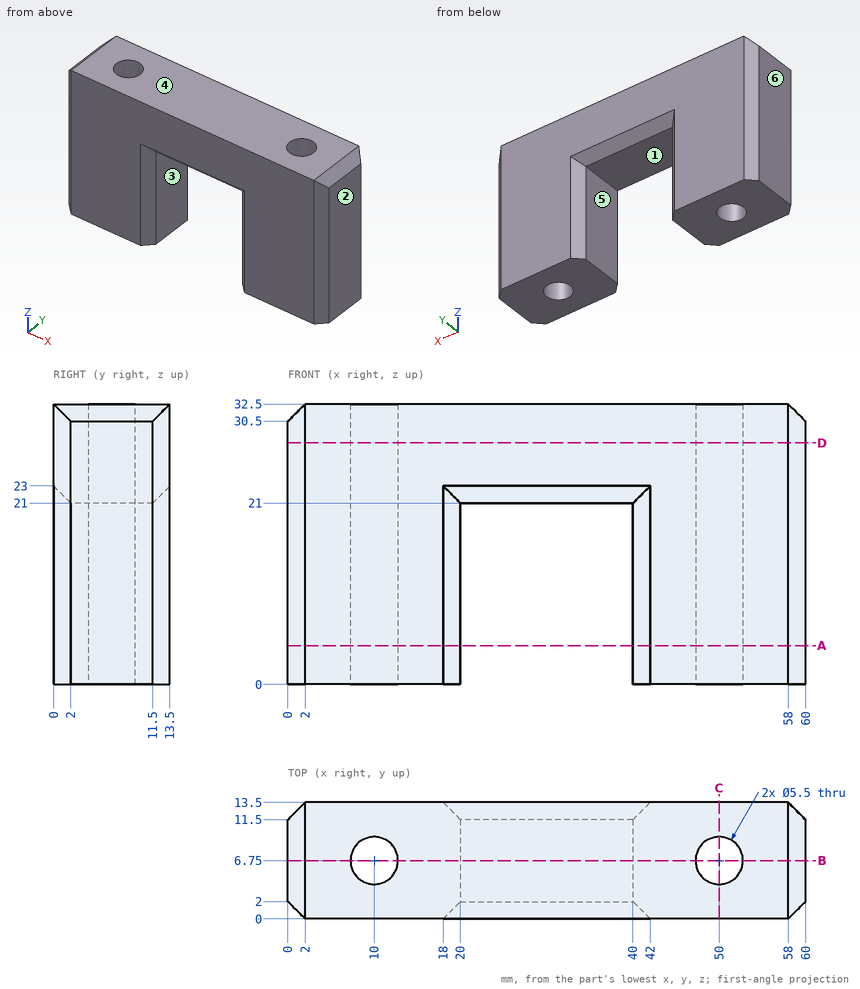
Job drawing, mm, ordinate dimensions from the low corner. One solid piece. A direction names the side the tool comes from. Coordinates: 2 decimals unless noted, no trailing zeros. Order: outer loops, then holes, each group sorted by start corner. A loop starts at its lowest first (then second) coordinate and runs counter-clockwise, first axis right, second up. Notation, with made-up numbers: (43, 9.25) -> (48, 9.25) arc R11 ccw to (48, 21.25) -> close; hole circle Ø8 at (-23, -34.5). An arc over 180 degrees is marked (long way). Put each result on its own line as item: value. Start each with the question number.
(1) Band-saw the part on B-B (y = 6.75). Give the cut face in (x, z), then the cut area to 3 significant figures.
(2) Pin check, flat tip, straight feed: pin 1 Ø1 at (x, y) = (30, 4) entering from -Z. Stop position of the tip, or through.
(3) Band-saw the part on D-D (z = 28). Give the cut face in (x, y), then the cut area to 3 significant figures.
(4) Band-saw the part on A-A (z = 4.5). Give the cut face in (x, y).
(5) Mould opens along X. For the marked faces 3, 4, 5 and 6 say: pulls with the +X half, pulls with the -X half, needs draft (parallel to the pull), parting line crosses it, or undercut.
(6) Which spindle directions (+Z, -Z, +X, -X, +Y, -Y) get a long thin tool onto all of the face, cutting with end or side? Do the marked faces 1 and 2. Say none if no direction does.
(7) Band-saw the part on C-C (x = 50). Give the cut face in (y, z).
(8) Probe line 1 along X through (y, z) = (7, 5); line 2 along X through (y, z) = (7.25, 27.5); line 3 along X through (y, z) = (4.5, 22.5). List the from-to ranges inside material, lowest first. Write a range as [from, to].
Determined:
1. outline: (0, 0) -> (7.25, 0) -> (7.25, 32.5) -> (2, 32.5) -> (0, 30.5) -> close; (12.75, 0) -> (20, 0) -> (20, 21) -> (40, 21) -> (40, 0) -> (47.25, 0) -> (47.25, 32.5) -> (12.75, 32.5) -> close; (52.75, 0) -> (60, 0) -> (60, 30.5) -> (58, 32.5) -> (52.75, 32.5) -> close
1. area: 1,170 mm²
2. pin 1: stops at z = 21
3. outline: (0, 2) -> (2, 0) -> (58, 0) -> (60, 2) -> (60, 11.5) -> (58, 13.5) -> (2, 13.5) -> (0, 11.5) -> close; hole circle Ø5.5 at (10, 6.75); hole circle Ø5.5 at (50, 6.75)
3. area: 754 mm²
4. outline: (0, 2) -> (2, 0) -> (18, 0) -> (20, 2) -> (20, 11.5) -> (18, 13.5) -> (2, 13.5) -> (0, 11.5) -> close; (40, 2) -> (42, 0) -> (58, 0) -> (60, 2) -> (60, 11.5) -> (58, 13.5) -> (42, 13.5) -> (40, 11.5) -> close; hole circle Ø5.5 at (10, 6.75); hole circle Ø5.5 at (50, 6.75)
5. face 3: undercut
5. face 4: needs draft
5. face 5: undercut
5. face 6: pulls with the -X half
6. face 1: -Z, +Y, -Y
6. face 2: +Z, -Z, +X, +Y, -Y
7. outline: (0, 0) -> (4, 0) -> (4, 32.5) -> (0, 32.5) -> close; (9.5, 0) -> (13.5, 0) -> (13.5, 32.5) -> (9.5, 32.5) -> close
8. line 1: x = [0, 7.26], [12.74, 20], [40, 47.26], [52.74, 60]
8. line 2: x = [0, 7.3], [12.7, 47.3], [52.7, 60]
8. line 3: x = [0, 8.42], [11.58, 48.42], [51.58, 60]
